Autodesk Inventor part; units mm, degrees
ref_plane "YZ Plane" through (0, 0, 0) normal (1, 0, 0) x (0, 1, 0)
ref_plane "XZ Plane" through (0, 0, 0) normal (0, 1, 0) x (-1, 0, 0)
ref_plane "XY Plane" through (0, 0, 0) normal (0, 0, 1) x (1, 0, 0)
sketch "Sketch1" plane through (0, 0, 0) normal (0, 0, 1) x (1, 0, 0)
  line L0 (-96.9802, 31.1578) -> (83.0198, 31.1578)
  line L1 (83.0198, 31.1578) -> (83.0198, -28.8422)
  line L2 (83.0198, -28.8422) -> (-96.9802, -28.8422)
  line L3 (-96.9802, -28.8422) -> (-96.9802, 31.1578)
  point P0 (0, 0)
  dimension "d0" = 180
  dimension "d1" = 60
extrude "Extrusion1" add sketch "Sketch1" along normal blind 10
sketch "Sketch4" plane through (0, 0, 0) normal (0, 0, -1) x (-1, 0, 0)
  circle A0 centre (-21.0198, -7.6922) radius 11.5
  line L0 (96.9802, -28.8422) -> (-83.0198, -28.8422)
  line L1 (-83.0198, -28.8422) -> (-83.0198, 31.1578)
  point P0 (0, 0)
  dimension "d16" = 23
  dimension "d17" = 21.15
  dimension "d18" = 62
extrude "Extrusion4" cut sketch "Sketch4" against normal through all
sketch "Sketch5" plane through (0, 0, 0) normal (0, 0, -1) x (-1, 0, 0)
  line L0 (96.9802, -28.8422) -> (-83.0198, -28.8422)
  line L1 (96.9802, 31.1578) -> (96.9802, -28.8422)
  line L2 (-83.0198, -28.8422) -> (96.9802, -28.8422)
  line L3 (96.9802, -28.8422) -> (96.9802, -22.8422)
  line L4 (96.9802, -22.8422) -> (-83.0198, -22.8422)
  line L5 (-83.0198, -22.8422) -> (-83.0198, -28.8422)
  point P0 (0, 0)
  dimension "d21" = 6
extrude "Extrusion5" add sketch "Sketch5" along normal blind 16
sketch "Sketch6" plane through (-96.9802, -22.8422, 0) normal (0, 1, 0) x (1, 0, 0)
  line L0 (180, 16) -> (0, 16)
  line L1 (180, 0) -> (0, 0)
  line L2 (165.9, 16) -> (159.9, 16)
  line L3 (159.9, 16) -> (159.9, 0)
  line L4 (159.9, 0) -> (165.9, 0)
  line L5 (165.9, 0) -> (165.9, 16)
  line L6 (14.1, 16) -> (20.1, 16)
  line L7 (20.1, 16) -> (20.1, 0)
  line L8 (20.1, 0) -> (14.1, 0)
  line L9 (14.1, 0) -> (14.1, 16)
  line L10 (0, 0) -> (0, 16)
  line L11 (180, 0) -> (180, 16)
  point P0 (96.9802, 0)
  point P1 (14.1, 16)
  point P2 (14.1, 0)
  point P3 (20.1, 16)
  point P4 (165.9, 0)
  dimension "d24" = 14.1
  dimension "d25" = 6
  dimension "d26" = 14.1
  dimension "d27" = 6
extrude "Extrusion6" add sketch "Sketch6" along normal blind 20 contours L5 L1 L3 L0 | L7 L1 L9 L0
sketch "Sketch7" plane through (-76.8802, -22.8422, 0) normal (0, 1, 0) x (1, 0, 0)
  line L0 (0, 16) -> (139.8, 16)
  line L1 (0, 16) -> (0, 0)
  line L2 (139.8, 16) -> (0, 16)
  line L3 (0, 16) -> (0, 0)
  line L4 (0, 0) -> (139.8, 0)
  line L5 (139.8, 0) -> (139.8, 16)
  point P0 (76.8802, 0)
extrude "Extrusion7" cut sketch "Sketch7" against normal through all
chamfer "Chamfer1" distance 3 angle 45 2 edges at (62.9198, -28.8422, -8) (-76.8802, -28.8422, -8)
sketch "Sketch8" plane through (0, 0, 10) normal (0, 0, 1) x (1, 0, 0)
  circle A0 centre (-34.9802, -7.6922) radius 11.05
  line L0 (-96.9802, -28.8422) -> (83.0198, -28.8422)
  line L1 (-96.9802, 31.1578) -> (-96.9802, -28.8422)
  point P0 (0, 0)
  dimension "d35" = 22.1
  dimension "d36" = 21.15
  dimension "d37" = 62
extrude "Extrusion8" cut sketch "Sketch8" against normal through all
chamfer "Chamfer2" distance 1 angle 45 2 edges at (-46.0302, -7.6922, 10) (-46.0302, -7.6922, 0)
sketch "Sketch9" plane through (-96.9802, -28.8422, 10) normal (0, -1, 0) x (1, 0, 0)
  circle A0 centre (10, -18) radius 2
  circle A1 centre (170, -18) radius 2
  line L0 (180, -26) -> (180, 0)
  line L1 (0, 0) -> (0, -26)
  line L2 (17.1, -26) -> (0, -26)
  line L3 (180, -26) -> (162.9, -26)
  point P0 (96.9802, -10)
  dimension "d43" = 4
  dimension "d44" = 10
  dimension "d45" = 4
  dimension "d46" = 10
  dimension "d47" = 8
  dimension "d48" = 8
extrude "Extrusion9" cut sketch "Sketch9" against normal through all
chamfer "Chamfer3" distance 3.5 angle 45 2 edges at (71.0198, -28.8422, -8) (-88.9802, -28.8422, -8)
sketch "Sketch10" plane through (0, 0, 10) normal (0, 0, 1) x (1, 0, 0)
  circle A0 centre (-86.9802, 25.1578) radius 1.5
  circle A1 centre (-51.9802, 25.1578) radius 1.5
  circle A2 centre (-6.9802, 25.1578) radius 1.5
  circle A3 centre (38.0198, 25.1578) radius 1.5
  circle A4 centre (73.0198, 25.1578) radius 1.5
  line L0 (83.0198, 31.1578) -> (-96.9802, 31.1578)
  line L1 (83.0198, -28.8422) -> (83.0198, 31.1578)
  line L2 (-96.9802, 31.1578) -> (-96.9802, -28.8422)
  point P0 (0, 0)
  dimension "d54" = 3
  dimension "d55" = 3
  dimension "d56" = 3
  dimension "d57" = 3
  dimension "d58" = 3
  dimension "d59" = 6
  dimension "d60" = 6
  dimension "d61" = 6
  dimension "d62" = 6
  dimension "d63" = 6
  dimension "d64" = 10
  dimension "d65" = 10
  dimension "d66" = 35
  dimension "d67" = 35
  dimension "d68" = 90
extrude "Extrusion10" cut sketch "Sketch10" against normal through all
chamfer "Chamfer4" distance 1.8 angle 45 5 edges at (-88.4802, 25.1578, 10) (-53.4802, 25.1578, 10) (-8.4802, 25.1578, 10) (36.5198, 25.1578, 10) (71.5198, 25.1578, 10)
sketch "Sketch11" plane through (-96.9802, -22.8422, -16) normal (-1, 0, 0) x (0, 0, 1)
  circle A0 centre (8, 10) radius 2
  line L0 (16, 0) -> (0, 0)
  line L1 (0, 0) -> (0, 20)
  point P0 (16, 22.8422)
  dimension "d77" = 4
  dimension "d78" = 10
  dimension "d79" = 8
extrude "Extrusion11" cut sketch "Sketch11" against normal through all
chamfer "Chamfer6" distance 3 angle 45 2 edges at (62.9198, -12.8422, -10) (-76.8802, -12.8422, -10)
sketch "Sketch12" plane through (0, 0, 0) normal (0, 0, -1) x (-1, 0, 0)
  circle A0 centre (-36.5198, 7.8078) radius 1.5
  circle A1 centre (-5.5198, 7.8078) radius 1.5
  circle A2 centre (-5.5198, -23.1922) radius 1.5
  circle A3 centre (-36.5198, -23.1922) radius 1.5
  circle A4 centre (-21.0198, -7.6922) radius 11.5
  point P0 (0, 0)
  dimension "d85" = 3
  dimension "d86" = 3
  dimension "d87" = 3
  dimension "d88" = 3
  dimension "d89" = 15.5
  dimension "d90" = 15.5
  dimension "d91" = 15.5
  dimension "d93" = 15.5
  dimension "d94" = 15.5
  dimension "d95" = 15.5
  dimension "d96" = 31
  dimension "d97" = 15.5
extrude "Extrusion12" cut sketch "Sketch12" against normal through all contours A0 | A1 | A2 | A3
chamfer "Chamfer7" distance 1.8 angle 45 4 edges at (38.0198, 7.8078, 0) (7.0198, 7.8078, 0) (7.0198, -23.1922, 0) (38.0198, -23.1922, 0)
sketch "Sketch13" plane through (-96.9802, -22.8422, -16) normal (-1, 0, 0) x (0, 0, 1)
  line L0 (16, 0) -> (16, 54)
  line L1 (16, 41.9) -> (21.1, 41.9)
  line L2 (21.1, 41.9) -> (21.1, 54)
  line L3 (21.1, 54) -> (16, 54)
  line L4 (16, 54) -> (16, 41.9)
  line L5 (26, 54) -> (16, 54)
  point P0 (16, 22.8422)
  point P1 (16, 52)
  point P2 (16, 52)
  dimension "d103" = 12.1
  dimension "d104" = 12.1
  dimension "d105" = 5.1
extrude "Extrusion13" cut sketch "Sketch13" against normal through all
sketch "Sketch14" plane through (68.9198, -22.8422, 0) normal (1, 0, 0) x (0, 0, -1)
  line L0 (16, 20) -> (0, 20)
  line L1 (0, 0) -> (16, 0)
  line L2 (0, 20) -> (16, 20)
  line L3 (16, 20) -> (16, 0)
  line L4 (16, 0) -> (0, 0)
  line L5 (0, 0) -> (0, 20)
  point P0 (0, 22.8422)
  point P1 (16, 20)
  point P2 (0, 0)
extrude "Extrusion14" cut sketch "Sketch14" against normal through all
sketch "Sketch15" plane through (83.0198, -28.8422, 10) normal (1, 0, 0) x (0, 0, -1)
  line L0 (0, 60) -> (0, 0)
  line L1 (0, 0) -> (26, 0)
  line L2 (26, 0) -> (26, 26.1)
  line L3 (26, 26.1) -> (0, 26.1)
  line L4 (0, 26.1) -> (0, 0)
  line L5 (10, 6) -> (26, 6)
  point P0 (10, 28.8422)
  point P1 (0, 26.1)
  dimension "d110" = 20.1
  dimension "d111" = 26
extrude "Extrusion15" add sketch "Sketch15" along normal blind 6
chamfer "Chamfer8" distance 6 angle 45 1 edges at (83.0198, -2.7422, 5)
chamfer "Chamfer9" distance 3 angle 45 1 edges at (89.0198, -28.8422, -3)
sketch "Sketch16" plane through (89.0198, -28.8422, 10) normal (1, 0, 0) x (0, 0, -1)
  circle A0 centre (18, 16.1) radius 2
  line L0 (26, 26.1) -> (10, 26.1)
  line L1 (26, 0) -> (26, 26.1)
  point P0 (10, 28.8422)
  point P1 (23, 26.1)
  dimension "d123" = 4
  dimension "d124" = 10
  dimension "d125" = 8
extrude "Extrusion16" cut sketch "Sketch16" against normal through all
chamfer "Chamfer11" distance 3.8 angle 45 1 edges at (89.0198, -12.7422, -6)
chamfer "Chamfer12" distance 6 angle 45 1 edges at (86.0198, -2.7422, -16)
sketch "Sketch17" plane through (-96.9802, -28.8422, 10) normal (-1, 0, 0) x (0, 0, 1)
  line L0 (0, 0) -> (-26, 0)
  line L1 (0, 0) -> (-26, 0)
  line L2 (-26, 0) -> (-26, 26.1)
  line L3 (-26, 26.1) -> (0, 26.1)
  line L4 (0, 26.1) -> (0, 0)
  point P0 (-10, 28.8422)
  dimension "d134" = 26
  dimension "d135" = 26.1
extrude "Extrusion17" add sketch "Sketch17" along normal blind 6
chamfer "Chamfer13" distance 6 angle 45 1 edges at (-96.9802, -2.7422, 5)
chamfer "Chamfer14" distance 3 angle 45 1 edges at (-102.9802, -28.8422, -3)
chamfer "Chamfer15" distance 6 angle 45 1 edges at (-99.9802, -2.7422, -16)
sketch "Sketch18" plane through (-102.9802, -28.8422, 10) normal (-1, 0, 0) x (0, 0, 1)
  circle A0 centre (-18, 16.1) radius 2
  circle A1 centre (-18, 16.1) radius 2
  point P0 (-10, 28.8422)
extrude "Extrusion18" cut sketch "Sketch18" against normal through all
chamfer "Chamfer16" distance 3.5 angle 45 1 edges at (-102.9802, -12.7422, -10)
sketch "Sketch19" plane through (0, 0, 10) normal (0, 0, 1) x (1, 0, 0)
  circle A0 centre (-86.9802, -12.8422) radius 2.7
  circle A1 centre (73.0198, -12.8422) radius 2.7
  line L0 (-96.9802, 31.1578) -> (-96.9802, 3.2578)
  line L1 (86.0198, -28.8422) -> (-99.9802, -28.8422)
  line L2 (83.0198, 3.2578) -> (83.0198, 31.1578)
  point P0 (0, 0)
  dimension "d152" = 5.4
  dimension "d153" = 5.4
  dimension "d154" = 10
  dimension "d155" = 16
  dimension "d156" = 10
  dimension "d157" = 16
extrude "Extrusion19" cut sketch "Sketch19" against normal through all
sketch "Sketch20" plane through (0, 0, -16) normal (0, 0, -1) x (-1, 0, 0)
  line L0 (102.9802, -2.7422) -> (96.9802, -2.7422)
  line L1 (-83.2198, -23.0422) -> (97.1802, -23.0422)
  line L2 (97.1802, -23.0422) -> (97.1802, -2.7422)
  line L3 (97.1802, -2.7422) -> (-83.2198, -2.7422)
  line L4 (-83.2198, -2.7422) -> (-83.2198, -23.0422)
  line L5 (96.9802, -8.7422) -> (96.9802, -22.8422)
  line L6 (96.9802, -22.8422) -> (76.8802, -22.8422)
  line L7 (-83.0198, -22.8422) -> (-83.0198, -8.7422)
  point P0 (0, 0)
  dimension "d164" = 0.2
  dimension "d165" = 0.2
  dimension "d166" = 0.2
extrude "Extrusion20" cut sketch "Sketch20" against normal up to surface (16 mm away)
chamfer "Chamfer18" distance 3 angle 45 2 edges at (-89.6802, -12.8422, 10) (70.3198, -12.8422, 10)
properties part number "wall" material "ABS Plastic"
The listing builds one solid part. Answer for the finished solid, in the listing's coordinates (mm). A direction names the side the tool comes from. Give positions to 0.01 mm unless a question says otherwise; leave off trailing zeros. Loops run counter-clockwise (first coordinate to the right, second up) from the corner with the lowest first, then second, coordinate; pieces in that order, holes last. Notation, with made-up numbers: (-4, 73) - (32, 73) arc R22 ccw to (32, 90) - close; hole circle Ø1 at (-10, 75). An arc over 180 degrees is marked (long way). Answer as a JSON object with one key per item and string values.
1. A cutting plane is placed at A-A (x = 27). Write down the section's boundary in (y, z) (3 decimals), then the cut area to 3 significant figures.
Determined:
{"outline": "(-28.842, 0) - (-17.515, 0) - (-17.515, 10) - (-28.842, 10) - close; (2.131, 0) - (19.058, 0) - (19.058, 5.1) - (31.158, 5.1) - (31.158, 10) - (2.131, 10) - close", "area": "342 mm²"}
2. For a pull along Y with two mould halves and no side action, classify faces 3 (the conical face through (71.74, 24.18, 8.31)), 4 (the flat face through (83.02, 14, 6)), 5 (the flat face through (85.978, 0.3, 4.93)) as pulls with the +Y half, pulls with the -Y half, needs draft (parallel to the pull), parting line crosses it, or undercut.
Determined:
{"face 3": "undercut", "face 4": "needs draft", "face 5": "pulls with the +Y half"}
3. For faces 1 (the flat face through (86.08, -5.78, -13.04)), 2 (the flat face through (-97.18, -15, -8)), determine the directions among +Z, -Z, +X, -X, +Y, -Y from which every point of the face is accessible in a straight line to the end or side of a thin tool.
Determined:
{"face 1": "-Z, +X, -X, +Y", "face 2": "-Z, +Y"}
4. A cutting plane is placed at B-B (z = -8). Give the number of separate pieces and of enclosed holes in the cut face, then the cut area to 3 significant figures.
Determined:
{"separate pieces": "6", "enclosed holes": "0", "area": "376 mm²"}
5. Flat-ended cylindrical pins translate along their axes: pin 1 Ø2.5 at (x, z) = (-86.98, -8) entering from -Y; pin 2 Ø6.5 at (y, z) = (-12.74, -8) entering from +X; pin 3 Ø10 at (x, z) = (9.5, -4.5) entering from +Y; pin 4 Ø3 at (x, z) = (-100, 0) entering from +Y. Find the tip coordinate at first contact, or state that the pin passes through.
Determined:
{"pin 1": "through", "pin 2": "x = 86.47", "pin 3": "y = 19.06", "pin 4": "y = 1.74"}
6. A cutting plane is placed at D-D (x = 0.5). Write down the section's boundary in (y, z), then the cut area to 3 significant figures.
Determined:
{"outline": "(-28.84, 0) - (19.06, 0) - (19.06, 5.1) - (31.16, 5.1) - (31.16, 10) - (-28.84, 10) - close", "area": "538 mm²"}
7. A cutting plane is placed at C-C (y = 15). Write down the section's boundary in (x, z).
Determined:
{"outline": "(-96.98, 0) - (83.02, 0) - (83.02, 10) - (-96.98, 10) - close"}
8. Find the intervals of material crossed by L1, parallel to Y at x = 83.7, z = -8; L2, parallel to X at y = -25.5, z = 0.75; L3, parallel to X at y = 5.5, z = 0.25, in increasing order. Write a range as [from, to].
Determined:
{"L1": "[-28.84, -14.74], [-10.74, -2.74]", "L2": "[-102.98, 4.44], [6.6, 35.44], [37.6, 89.02]", "L3": "[-96.98, 3.53], [7.51, 34.53], [38.51, 83.02]"}
